For this review, take the finished solid that the model builds, in its own axes (mm). A direction names the side the tool comes from. Coordinates: 2 decimals unless noted, no trailing zeros. Write each loop counter-clockwise with the first axis right and the second up, starting at its lowest first coordinate (ties: lowest second). Pieces come first, ordered by that corner, then holes.
```python
from build123d import *

# Parameters (mm, degrees)
BOSS_EXTRUDE2_DEPTH = 2.5


with BuildPart() as part:
    # Glass_Sketch → Boss-Extrude2 (new body)
    with BuildSketch(Plane.XY):
        with BuildLine():
            Line((-10.296075652, -23.145089286), (-10.296075652, 2.854910714))
            ThreePointArc((-10.296075652, 2.854910714), (-9.270949386, 5.329784448), (-6.796075652, 6.354910714))
            Line((-6.796075652, 6.354910714), (19.203924348, 6.354910714))
            ThreePointArc((19.203924348, 6.354910714), (21.678798083, 5.329784448), (22.703924348, 2.854910714))
            Line((22.703924348, 2.854910714), (22.703924348, 1.854910714))
            ThreePointArc((22.703924348, 1.854910714), (22.850370958, 1.501357324), (23.203924348, 1.354910714))
            Line((23.203924348, 1.354910714), (26.203924348, 1.354910714))
            ThreePointArc((26.203924348, 1.354910714), (28.678798083, 0.329784448), (29.703924348, -2.145089286))
            Line((29.703924348, -2.145089286), (29.703924348, -18.145089286))
            ThreePointArc((29.703924348, -18.145089286), (28.678798083, -20.61996302), (26.203924348, -21.645089286))
            Line((26.203924348, -21.645089286), (23.203924348, -21.645089286))
            ThreePointArc((23.203924348, -21.645089286), (22.850370958, -21.791535895), (22.703924348, -22.145089286))
            Line((22.703924348, -22.145089286), (22.703924348, -23.145089286))
            ThreePointArc((22.703924348, -23.145089286), (21.678798083, -25.61996302), (19.203924348, -26.645089286))
            Line((19.203924348, -26.645089286), (-6.796075652, -26.645089286))
            ThreePointArc((-6.796075652, -26.645089286), (-9.270949386, -25.61996302), (-10.296075652, -23.145089286))
        make_face()
    extrude(amount=BOSS_EXTRUDE2_DEPTH)


solid = part.part
```
1) Clearance check with flat-ended pins moving along their axes: P1, Ø1.1, axis at y = 2.5, z = 2, coming from the +X side; P2, Ø1, axis at y = -0.5, z = 1, coming from the +X side. State where each tip first meets the part, or that it passes through.
2) Tool access review of faces 1 (the face through (6, -26.645, 1)), 2 (the face through (25, 1.355, 1)), 3 (the face through (25, -21.645, 1)): name each direction out of +Z, -Z, +X, -X, +Y, -Y from which nothing blocks a thin tool from reaching the whole face with its end or side.
3) For L1, parallel to X at y = 2, z = 0.35; L2, parallel to Y at x = -8, z = 0.1; L3, parallel to X at y = 0.5, z = 1.5, list the stretches that pass through material, from the lowest coordinate up.
4) Consider section A-A (z = 0.7). Give the boundary of the cut face in (x, y), then the cut area to 3 significant figures.
5) Consider section C-C (y = 4.5). Give the boundary of the cut face in (x, z).
6) Consider section B-B (x = 27). Give the boundary of the cut face in (y, z).
Results:
1. P1: stops at x = 22.7
1. P2: stops at x = 29.51
2. face 1: +Z, -Z, +X, -X, -Y
2. face 2: +Z, -Z, +X, +Y
2. face 3: +Z, -Z, +X, -Y
3. L1: x = -10.3 to 22.7
3. L2: y = -26.43 to 6.14
3. L3: x = -10.3 to 28.5
4. outline: (-10.3, -23.15) arc R3.5 ccw to (-6.8, -26.65) - (19.2, -26.65) arc R3.5 ccw to (22.7, -23.15) - (22.7, -22.15) arc R0.5 cw to (23.2, -21.65) - (26.2, -21.65) arc R3.5 ccw to (29.7, -18.15) - (29.7, -2.15) arc R3.5 ccw to (26.2, 1.35) - (23.2, 1.35) arc R0.5 cw to (22.7, 1.85) - (22.7, 2.85) arc R3.5 ccw to (19.2, 6.35) - (-6.8, 6.35) arc R3.5 ccw to (-10.3, 2.85) - close
4. area: 1,230 mm2
5. outline: (-9.89, 0) - (22.29, 0) - (22.29, 2.5) - (-9.89, 2.5) - close
6. outline: (-21.55, 0) - (1.26, 0) - (1.26, 2.5) - (-21.55, 2.5) - close
